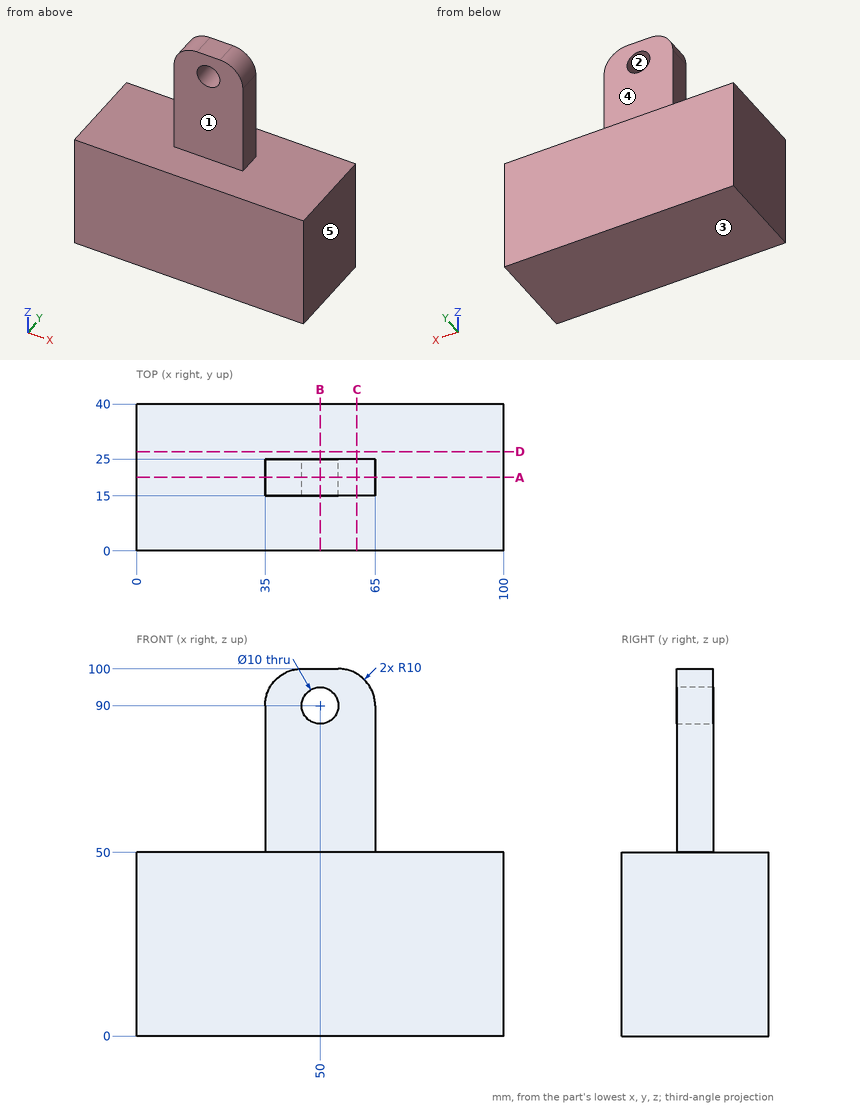
Can you work these out from the drawing? Everything is in mm from the part's minimum corner. A direction names the side the tool comes from. Coordinates: 2 decimals unless noted, no trailing zeros. Write each loop counter-clockwise with the first axis right and the second up, starting at its lowest first coordinate (ties: lowest second). Pieces come first, ordered by that corner, then holes. Notation, with made-up numbers: (-2.5, 22) - (52.5, 22) arc R18 cw to (52.5, 47) - close; hole circle Ø10 at (31, 27.5). An arc over 180 degrees is marked (long way). Use a Markdown table: item, result.
Q1. Please list where these lines run through material, in increasing order: L1, parallel to X at y = 18.5, z = 90; L2, parallel to Y at x = 47, z = 78; L3, parallel to Z at x = 32, y = 29.5.
Geometry check:
| item | result |
|---|---|
| L1 | x = 35 to 45, 55 to 65 |
| L2 | y = 15 to 25 |
| L3 | z = 0 to 50 |
Q2. Imagine slicing it at D-D (y = 27). List the corners of the cut face in (x, z) for me, and give its area (3 significant figures).
Geometry check:
| item | result |
|---|---|
| outline | (0, 0) - (100, 0) - (100, 50) - (0, 50) - close |
| area | 5,000 mm2 |
Q3. Thinking about a two-plate mould opening in Z: for the marked faces 1, 2 and 3, which applies, +Z half, -Z half, draft (parallel to the pull), parting line (faces both ways), or undercut?
Geometry check:
| item | result |
|---|---|
| face 1 | draft |
| face 2 | undercut |
| face 3 | -Z half |
Q4. I'm going to push flat-ended pins straight in: pin 1 Ø5 at (y, z) = (20, 62) entering from +X; pin 2 Ø1.5 at (x, z) = (55.5, 74) entering from +Y; pin 3 Ø2 at (x, z) = (65, 56) entering from -Y. Where does each tip first touch, or does it pass through?
Geometry check:
| item | result |
|---|---|
| pin 1 | stops at x = 65 |
| pin 2 | stops at y = 25 |
| pin 3 | stops at y = 15 |
Q5. Imagine slicing it at A-A (y = 20). List the corners of the cut face in (x, z) for me.
Geometry check:
| item | result |
|---|---|
| outline | (0, 0) - (100, 0) - (100, 50) - (65, 50) - (65, 90) arc R10 ccw to (55, 100) - (45, 100) arc R10 ccw to (35, 90) - (35, 50) - (0, 50) - close; hole circle Ø10 at (50, 90) |
Q6. Imagine slicing it at B-B (x = 50). List the corners of the cut face in (y, z) for me.
Geometry check:
| item | result |
|---|---|
| outline | (0, 0) - (40, 0) - (40, 50) - (25, 50) - (25, 85) - (15, 85) - (15, 50) - (0, 50) - close; (15, 95) - (25, 95) - (25, 100) - (15, 100) - close |
Q7. Imagine slicing it at C-C (x = 60). List the corners of the cut face in (y, z) for me, and give its area (3 significant figures).
Geometry check:
| item | result |
|---|---|
| outline | (0, 0) - (40, 0) - (40, 50) - (25, 50) - (25, 98.66) - (15, 98.66) - (15, 50) - (0, 50) - close |
| area | 2,490 mm2 |
Q8. Which directions (+Z, -Z, +X, -X, +Y, -Y) give clear straight access to the entire face, cutting with the end or side of a thin tool? Please do the marked faces 4 and 5.
Geometry check:
| item | result |
|---|---|
| face 4 | +Z, +X, -X, +Y |
| face 5 | +Z, -Z, +X, +Y, -Y |
